from build123d import *

# Parameters (mm, degrees)
SKETCH1_W           = 81.28
SKETCH1_H           = 101.6
BOSS_EXTRUDE1_DEPTH = 1.27
SKETCH2_W           = 58.42
SKETCH2_H           = 81.28
BOSS_EXTRUDE2_DEPTH = 27.94
FILLET1_R           = 2.54
SKETCH4_R           = 1
BOSS_EXTRUDE3_DEPTH = 11.43


with BuildPart() as part:
    # Sketch1 → Boss-Extrude1 (new body)
    with BuildSketch(Plane(origin=(0, 0, 0), x_dir=(1, 0, 0), z_dir=(0, 1, 0))):
        Rectangle(SKETCH1_W, SKETCH1_H)
    extrude(amount=BOSS_EXTRUDE1_DEPTH)

    # Sketch2 → Boss-Extrude2 (add)
    with BuildSketch(Plane(origin=(0, 1.27, 0), x_dir=(1, 0, 0), z_dir=(0, 1, 0))):
        with Locations((0.667132778, 0)):
            Rectangle(SKETCH2_W, SKETCH2_H)
    extrude(amount=BOSS_EXTRUDE2_DEPTH)

    # Fillet1
    fillet1_edges = [part.edges().sort_by_distance(p)[0] for p in [
        (40.64, 0.635, 50.8),
        (-40.64, 0.635, 50.8),
        (-40.64, 0.635, -50.8),
        (40.64, 0.635, -50.8),
    ]]
    fillet(fillet1_edges, radius=FILLET1_R)

    # Sketch4 → Boss-Extrude3 (add)
    with BuildSketch(Plane.XZ):
        with Locations((38.1, 48.26)):
            Circle(SKETCH4_R)
        with Locations((38.1, -48.26)):
            Circle(SKETCH4_R)
        with Locations((-38.1, 48.26)):
            Circle(SKETCH4_R)
        with Locations((-38.1, -48.26)):
            Circle(SKETCH4_R)
    extrude(amount=BOSS_EXTRUDE3_DEPTH)


solid = part.part
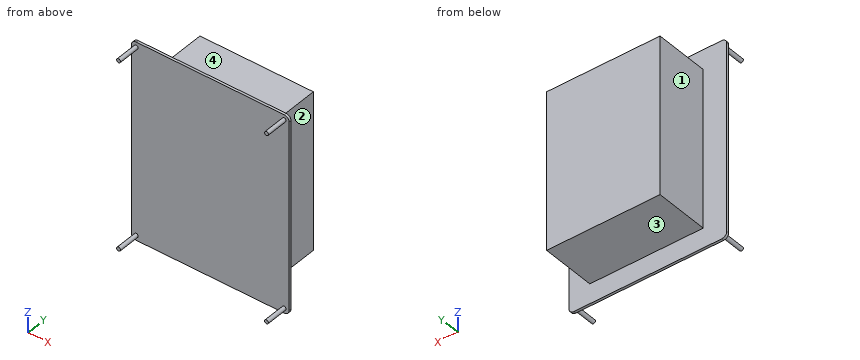
Input: part model. Units: mm. Frame: model coordinates. Face numbers are marked on the shaded views. A direction names the side the tool comes from. Give positions to 0.01 mm unless a question says otherwise; leave off trailing zeros. Write each loop counter-clockwise with the first axis right and the second up, starting at its lowest first coordinate (ties: lowest second). Pieces come first, ordered by that corner, then holes. Notation, with made-up numbers: (-16.75, 25) -> (-1.75, 25) arc R16 cw to (-1.75, 38) -> close; hole circle Ø11 at (58.25, 3). An arc over 180 degrees is marked (long way). Use one line per item in the form item = value. Start each with the question number.
1) Section query D-D on y = 7. Return the cut outline in (x, z), then the cut area to 3 significant figures.
2) Pin query (flat end, axial travel): pin 1 (1.5 mm diameter, centred on x = 21.5, y = 1.5, fed in from -Z); pin 2 (22.5 mm diameter, centred on y = 19, z = -12.5, fed in from -X); pin 3 (3 mm diameter, centred on x = -21, y = 12, fed in from +Z); pin 4 (8.5 mm diameter, centred on x = -5, y = 16.5, fed in from -Z). Return the tip coordinate at first contact, or that it passes through.
3) Set-up query: the marked faces 1, 2, 3 and 4. Return all of +Z, -Z, +X, -X, +Y, -Y with unobstructed straight access to the full face (end or side cutting, diameter ignored); none if empty.
4) Section query B-B on x = 19. Return the cut outline in (y, z).
5) Section query C-C on y = -2. Return the cut outline in (x, z).
6) Section query A-A on z = -31.5. Return the cut outline in (x, y).
7) Ray query, probe 1 along Y at (x, z) = (-35, -2.5); probe 2 along Y at (x, z) = (19.5, 12); probe 3 along X at (y, z) = (5.5, -28.5). Return the intervals inside material, ascending. Write a range as from..to.
Outcome:
q1.outline = (-28.54, -40.64) -> (29.88, -40.64) -> (29.88, 40.64) -> (-28.54, 40.64) -> close
q1.area = 4,750 mm^2
q2.pin_1 = -50.8
q2.pin_2 = -28.54
q2.pin_3 = 40.64
q2.pin_4 = -40.64
q3.face_1 = +Z, -Z, -X, +Y
q3.face_2 = +Z, -Z, +X, +Y
q3.face_3 = -Z, +X, -X, +Y
q3.face_4 = +Z, +X, -X, +Y
q4.outline = (0, -50.8) -> (1.27, -50.8) -> (1.27, -40.64) -> (29.21, -40.64) -> (29.21, 40.64) -> (1.27, 40.64) -> (1.27, 50.8) -> (0, 50.8) -> close
q5.outline = circle Ø2 at (-38.1, -48.26); circle Ø2 at (-38.1, 48.26); circle Ø2 at (38.1, -48.26); circle Ø2 at (38.1, 48.26)
q6.outline = (-40.64, 0) -> (40.64, 0) -> (40.64, 1.27) -> (29.88, 1.27) -> (29.88, 29.21) -> (-28.54, 29.21) -> (-28.54, 1.27) -> (-40.64, 1.27) -> close
q7.probe_1 = 0..1.27
q7.probe_2 = 0..29.21
q7.probe_3 = -28.54..29.88
